Model file for the job. Use its own axes, mm. A direction names the side the tool comes from. Coordinates: 2 decimals unless noted, no trailing zeros. Order: outer loops, then holes, each group sorted by start corner. A loop starts at its lowest first (then second) coordinate and runs counter-clockwise, first axis right, second up. Notation, with made-up numbers: (50, 48) -> (74, 48) arc R16 cw to (74, 69) -> close; hole circle Ø6 at (73, 24.25). An arc over 180 degrees is marked (long way). Use CSV: the item, a comma, the result in double quotes. Start each with the question number.
(1) Tool access for faces 4 (the flat face through (-5, 7.95, 5)), 5 (the flat face through (-6, -7.95, 5)), 6 (the flat face through (19, -4.085, 5)), 7 (the flat face through (19, 1.915, 5)): list every direction of +Z, -Z, +X, -X, +Y, -Y with a clear straight run to the whole face (end or side of a thin tool).
(2) Cut at B-B on y = -5.15. Write the cut outline in (x, z).
(3) Cut at C-C on z = 1. Give the number of separate pieces and of enclosed holes in the cut face, plus the area to 3 significant figures.
(4) Pull direction Y, two halves, no side cores. Call faces 1 (the flat face through (6, -10.42, 5)), 2 (the flat face through (0, 0, 10.3)), 3 (the flat face through (19, 2.65, 5)): pulls with the +Y half, pulls with the -Y half, needs draft (parallel to the pull), parting line crosses it, or undercut.
(5) Probe L1, parallel to X at y = 5.15, z = 7; L2, parallel to Y at x = 15.5, z = 1.75; L3, parallel to X at y = -5.15, z = 5. List the from-to ranges inside material, lowest first.
(6) Cut at A-A on x = -4.5. Write the cut outline in (y, z), plus the area to 3 significant figures.
(7) Pin check, flat tips, straight feed: pin 1 Ø4.5 at (x, z) = (5.5, 7) entering from +Y; pin 2 Ø4.5 at (x, z) = (5, 5) entering from +Y (3 decimals); pin 3 Ø1.3 at (y, z) = (-9, 7.5) entering from -X. Stop position of each tip, or through.
```python
from build123d import *

# Parameters (mm, degrees)
IZIM1_R                     = 1.5
Y_KSEKLIK_EKSTR_ZYON1_DEPTH = 10.3
RADYUS2_R                   = 2
IZIM4_R                     = 0.77
Y_KSEKLIK_EKSTR_ZYON2_DEPTH = 10.3


with BuildPart() as part:
    # Çizim1 → Yükseklik-Ekstrüzyon1 (new body)
    with BuildSketch(Plane.XY):
        with BuildLine():
            Line((13.9, -4.084784969), (22.330620506, -4.084784969))
            Line((22.330620506, -4.084784969), (23.3, -4.084784969))
            Line((23.3, -4.084784969), (23.3, -3.910005756))
            Line((23.3, -3.910005756), (23.3, -3.608421024))
            Line((23.3, -3.608421024), (23.3, -3.349919826))
            Line((23.3, -3.349919826), (22.330620506, -3.349919826))
            Line((22.330620506, -3.349919826), (13.9, -3.349919826))
            Line((13.9, -3.349919826), (13.9, 1.915215031))
            Line((13.9, 1.915215031), (22.330620506, 1.915215031))
            Line((22.330620506, 1.915215031), (23.3, 1.915215031))
            Line((23.3, 1.915215031), (23.3, 2.089994244))
            Line((23.3, 2.089994244), (23.3, 2.391578976))
            Line((23.3, 2.391578976), (23.3, 2.650080174))
            Line((23.3, 2.650080174), (22.330620506, 2.650080174))
            Line((22.330620506, 2.650080174), (13.9, 2.650080174))
            Line((13.9, 2.650080174), (13.9, 7.95))
            Line((13.9, 7.95), (3, 7.95))
            Line((3, 7.95), (3, 10.116757373))
            Line((3, 10.116757373), (-9.1, 10.116757373))
            Line((-9.1, 10.116757373), (-9.1, 10.886757373))
            ThreePointArc((-9.1, 10.886757373), (-9.6, 11.386757373), (-10.1, 10.886757373))
            Line((-10.1, 10.886757373), (-10.1, 9.386757373))
            Line((-10.1, 9.386757373), (-9.1, 9.386757373))
            Line((-9.1, 9.386757373), (2.27, 9.386757373))
            Line((2.27, 9.386757373), (2.27, 7.95))
            Line((2.27, 7.95), (-13.9, 7.95))
            Line((-13.9, 7.95), (-13.9, -7.95))
            Line((-13.9, -7.95), (1.014637994, -7.95))
            Line((1.014637994, -7.95), (1.014637994, -11.15))
            Line((1.014637994, -11.15), (11.1, -11.15))
            Line((11.1, -11.15), (11.1, -10.42))
            Line((11.1, -10.42), (1.744637994, -10.42))
            Line((1.744637994, -10.42), (1.744637994, -7.95))
            Line((1.744637994, -7.95), (13.9, -7.95))
            Line((13.9, -7.95), (13.9, -4.084784969))
        make_face()
        with Locations(Location((11.1, 5.15, 0), (0, 0, 180))):
            Circle(IZIM1_R, mode=Mode.SUBTRACT)
        with Locations(Location((-11.1, -5.15, 0), (0, 0, 180))):
            Circle(IZIM1_R, mode=Mode.SUBTRACT)
    extrude(amount=Y_KSEKLIK_EKSTR_ZYON1_DEPTH)

    # Radyus2
    radyus2_edges = [part.edges().sort_by_distance(p)[0] for p in [
        (1.014637994, -11.15, 5.15),
        (-13.9, -7.95, 5.15),
        (-13.9, 7.95, 5.15),
        (3, 10.116757373, 5.15),
        (13.9, 7.95, 5.15),
        (13.9, -7.95, 5.15),
    ]]
    fillet(radyus2_edges, radius=RADYUS2_R)

    # Çizim4 → Yükseklik-Ekstrüzyon2 (add)
    with BuildSketch(Plane.XY.offset(10.3)):
        with Locations((-9.6, 10.886757373)):
            Circle(IZIM4_R)
    extrude(amount=-Y_KSEKLIK_EKSTR_ZYON2_DEPTH)


solid = part.part
```
Outcome:
1,face 4,"+Z, -Z, -X"
1,face 5,"+Z, -Z, -X, -Y"
1,face 6,"+Z, -Z, +X, -Y"
1,face 7,"+Z, -Z, +X"
2,outline,"(-13.9, 0) -> (-12.6, 0) -> (-12.6, 10.3) -> (-13.9, 10.3) -> close; (-9.6, 0) -> (13.9, 0) -> (13.9, 10.3) -> (-9.6, 10.3) -> close"
3,separate pieces,"1"
3,enclosed holes,"2"
3,area,"458 mm2"
4,face 1,"undercut"
4,face 2,"needs draft"
4,face 3,"pulls with the +Y half"
5,L1,"-13.9 to 9.6, 12.6 to 13.9"
5,L2,"-4.08 to -3.35, 1.92 to 2.65"
5,L3,"-13.9 to -12.6, -9.6 to 13.9"
6,outline,"(-7.95, 0) -> (7.95, 0) -> (7.95, 10.3) -> (-7.95, 10.3) -> close; (9.39, 0) -> (10.12, 0) -> (10.12, 10.3) -> (9.39, 10.3) -> close"
6,area,"171 mm2"
7,pin 1,"y = 7.95"
7,pin 2,"y = 9.085"
7,pin 3,"x = 1.01"
